For this review, use the dimensioned drawing (mm, ordinates from the lowest corner) and the shaded views. Round coordinates to 2 decimals unless told otherwise and drop trailing zeros. Write each loop counter-clockwise with the first axis right and the second up, starting at its lowest first coordinate (ties: lowest second). Pieces come first, ordered by that corner, then holes. Notation, with made-up numbers: (59.25, -34.5) - (90.25, -34.5) arc R26 ccw to (90.25, -3.5) - close; hole circle Ø3 at (47.5, 45). An arc over 180 degrees is marked (long way). Return JSON: item names as keys, results as strings.
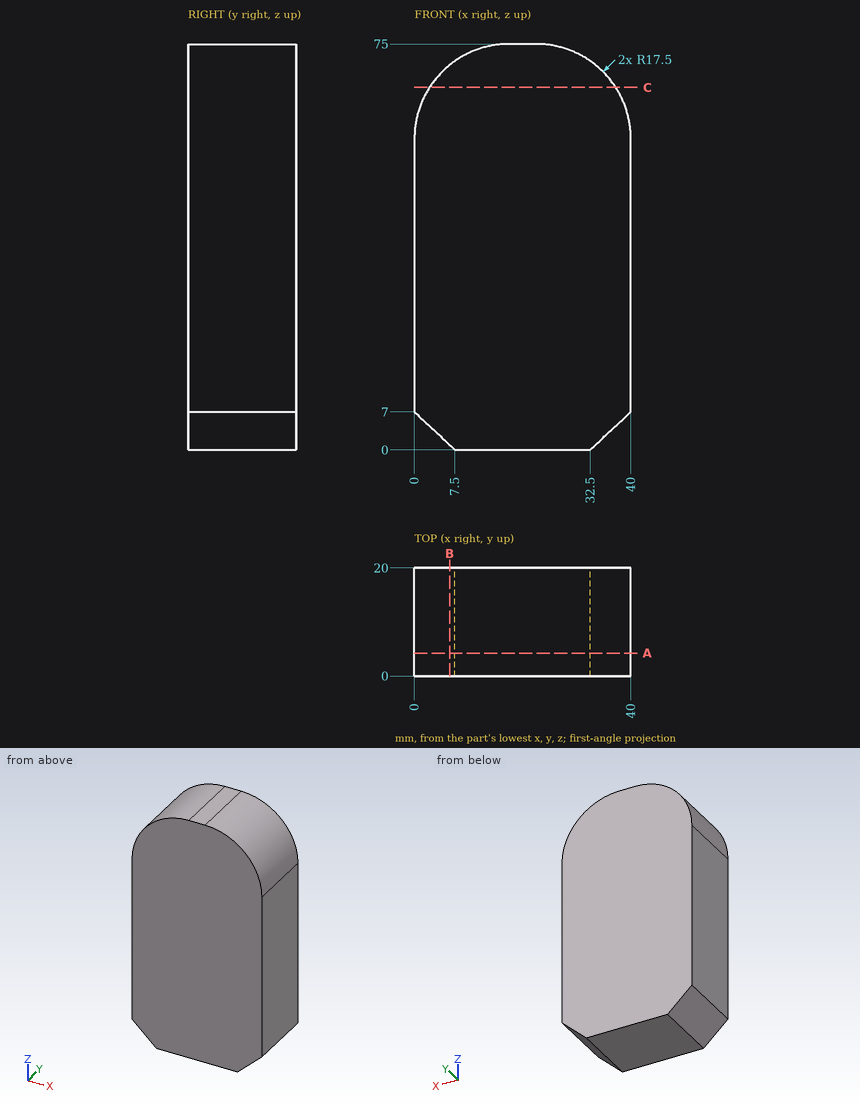
(1) Add section A-A (y = 4.25). Write out the cut boundary in (x, z), plus the area to 3 significant figures.
Filled in:
{"outline": "(0, 7) - (7.5, 0) - (32.5, 0) - (40, 7) - (40, 57.5) arc R17.5 ccw to (22.5, 75) - (17.5, 75) arc R17.5 ccw to (0, 57.5) - close", "area": "2,820 mm2"}
(2) Clearance check with a flat-ended pin moving along its axis: pin 1 Ø3 at (x, y) = (28, 10) entering from +Z. State where the tip first meets the part, or that it passes through.
Filled in:
{"pin 1": "stops at z = 74.54"}
(3) Wall thickness on line 1 (X direction, y = 5.5, z = 58); line 2 (Z direction, x = 14, y = 6.5); line 3 (X direction, y = 5, z = 63.5): over which ranges is each line inside the solid? List them lowest first.
Filled in:
{"line 1": "x = 0.01 to 39.99", "line 2": "z = 0 to 74.65", "line 3": "x = 1.06 to 38.94"}
(4) Add section C-C (z = 67). Write out the cut boundary in (x, y), plus the area to 3 significant figures.
Filled in:
{"outline": "(2.8, 0) - (37.2, 0) - (37.2, 20) - (2.8, 20) - close", "area": "688 mm2"}
(5) Add section B-B (x = 6.5). Write out the cut boundary in (y, z).
Filled in:
{"outline": "(0, 0.93) - (20, 0.93) - (20, 71.11) - (0, 71.11) - close"}
